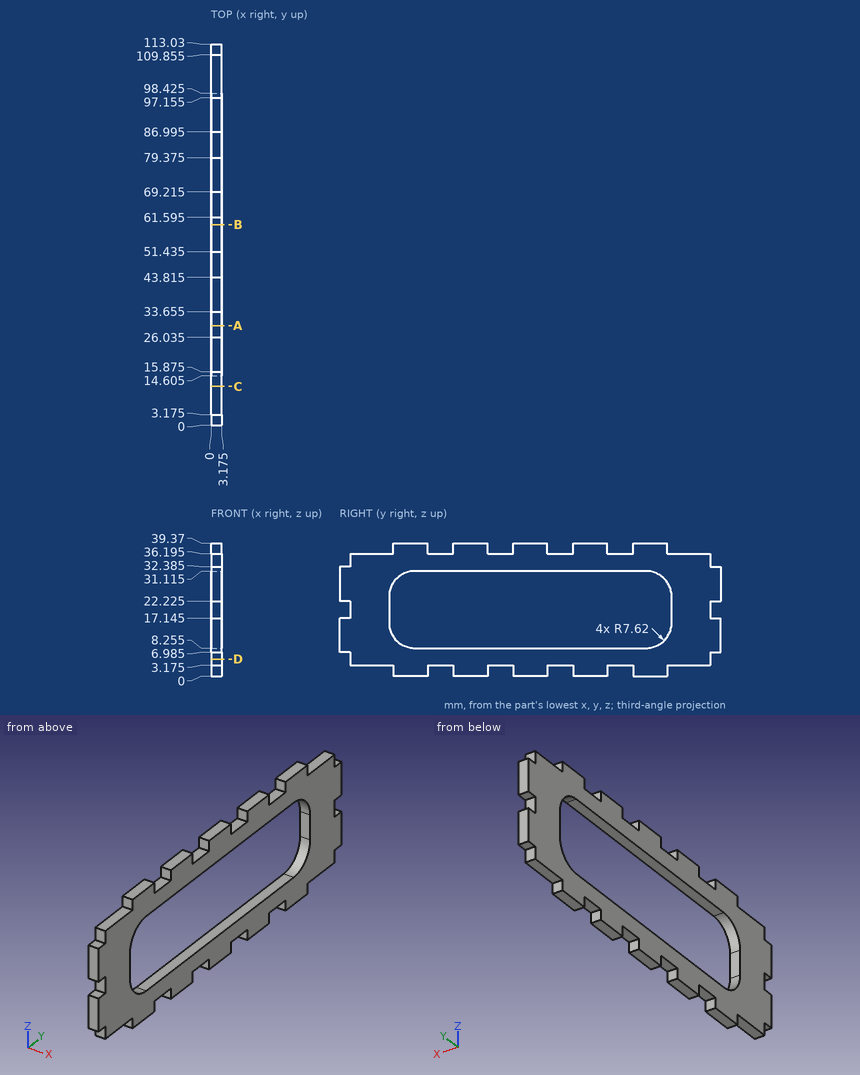
Can you work these out from the drawing? Everything is in mm from the part's minimum corner. Give positions to 0.01 mm unless a question says otherwise; leave off trailing zeros. Order: outer loops, then holes, each group sorted by start corner. A loop starts at its lowest first (then second) coordinate and runs counter-clockwise, first axis right, second up. Notation, with made-up numbers: M 80,29.25 L 98,29.25 A16 cw 98,56.25 Z; hole C 61.25,-9 d11. An arc over 180 degrees is marked long. Use a Markdown table: item, result. Add a question column.
1. Suppose I cut it at D-D (z = 5). List the corners of the cut face in (x, y) for me (3 decimals), and give its area (3 significant figures).
2. Suppose I cut it at B-B (y = 59.5). List the corners of the cut face in (x, z) for me (3 decimals).
3. I need wall thicknesses on probe 1 along Y at (x, z) = (2.1, 3) (3 decimals); probe 2 along Z at (x, y) = (2.8, 22); probe 3 along Z at (x, y) = (1.8, 30.5) (3 decimals). Which ranges of each line are inside material? Lowest first, please. Write a range as from..to.
4. For pin 1 Ø1.6 at (x, z) = (1, 37.5) entering from +Y (3 decimals); pin 2 Ø1.6 at (x, z) = (2, 5.5) entering from -Y (3 decimals); pin 3 Ø1 at (x, y) = (2.5, 83) entering from -Z (3 decimals), each with a flat end and sliding along its axis, tell me the tip position at first contact or that it passes through.
5. Suppose I cut it at A-A (y = 29.5). List the corners of the cut face in (x, z) for me (3 decimals), and give its area (3 significant figures).
6. Suppose I cut it at C-C (y = 11.5). List the corners of the cut face in (x, z) for me (3 decimals).
Results list:
| question | item | result |
|---|---|---|
| 1 | outline | M 0,3.175 L 3.175,3.175 L 3.175,109.855 L 0,109.855 Z |
| 1 | area | 339 mm² |
| 2 | outline | M 0,0 L 3.175,0 L 3.175,8.255 L 0,8.255 Z; M 0,31.115 L 3.175,31.115 L 3.175,39.37 L 0,39.37 Z |
| 3 | probe 1 | y = 15.875..26.035, 33.655..43.815, 51.435..61.595, 69.215..79.375, 86.995..97.155 |
| 3 | probe 2 | z = 0..8.26, 31.11..39.37 |
| 3 | probe 3 | z = 3.175..8.255, 31.115..36.195 |
| 4 | pin 1 | stops at y = 97.155 |
| 4 | pin 2 | stops at y = 3.175 |
| 4 | pin 3 | stops at z = 3.175 |
| 5 | outline | M 0,3.175 L 3.175,3.175 L 3.175,8.255 L 0,8.255 Z; M 0,31.115 L 3.175,31.115 L 3.175,36.195 L 0,36.195 Z |
| 5 | area | 32.3 mm² |
| 6 | outline | M 0,3.175 L 3.175,3.175 L 3.175,36.195 L 0,36.195 Z |
